```python
from build123d import *

# Parameters (mm, degrees)
SKETCH1_R           = 14.2875
BOSS_EXTRUDE1_DEPTH = 6.35
SKETCH2_R           = 3.3782
CUT_EXTRUDE1_DEPTH  = 7.35
CHAMFER1_SIZE       = 3.175


with BuildPart() as part:
    # Sketch1 → Boss-Extrude1 (new body)
    with BuildSketch(Plane(origin=(0, 0, 0), x_dir=(0, 0, -1), z_dir=(1, 0, 0))):
        with BuildLine():
            Line((0, 0), (0, 25.4))
            Line((0, 25.4), (28.110381264, 81.266707127))
            ThreePointArc((28.110381264, 81.266707127), (50.8, 95.25), (73.489618736, 81.266707127))
            Line((73.489618736, 81.266707127), (101.6, 25.4))
            Line((101.6, 25.4), (101.6, 0))
            Line((101.6, 0), (0, 0))
        make_face()
        with Locations((50.8, 69.85)):
            Circle(SKETCH1_R, mode=Mode.SUBTRACT)
    extrude(amount=BOSS_EXTRUDE1_DEPTH)

    # Sketch2 → Cut-Extrude1 (cut, through all)
    with BuildSketch(Plane(origin=(6.35, 0, 0), x_dir=(0, 0, -1), z_dir=(1, 0, 0))):
        with Locations((12.7, 12.7)):
            Circle(SKETCH2_R)
        with Locations((50.8, 12.7)):
            Circle(SKETCH2_R)
        with Locations((88.9, 12.7)):
            Circle(SKETCH2_R)
    extrude(amount=-CUT_EXTRUDE1_DEPTH, mode=Mode.SUBTRACT)

    # Chamfer1
    chamfer1_edges = [part.edges().sort_by_distance(p)[0] for p in [
        (3.175, 0, 0),
        (3.175, 0, -101.6),
    ]]
    chamfer(chamfer1_edges, length=CHAMFER1_SIZE)


solid = part.part
```
Input: part model. Units: mm. Frame: model coordinates. Round coordinates to 2 decimals unless told otherwise and drop trailing zeros. Loops run counter-clockwise (first coordinate to the right, second up) from the corner with the lowest first, then second, coordinate; pieces in that order, holes last. Notation, with made-up numbers: (-32.5, -34.75) - (-28.5, -34.75) arc R18 ccw to (-28.5, -0.75) - close; hole circle Ø10 at (16, -39). An arc over 180 degrees is marked (long way). One line per item, written item: value. Start each with the question number.
(1) Contact query for flat-ended pins moving along their axis: P1, Ø3, axis at x = 1, z = -57.5, coming from the +Y side; P2, Ø2, axis at x = 4.5, z = -35.5, coming from the +Y side. Output: stop coordinate, or through.
(2) Section C-C, the plane x = 5. Count the separate pieces of the cut face and the enclosed holes in it, plus the area to 3 significant figures.
(3) Ray query, line 1 (Y direction, x = 3.25, z = -50.8); line 2 (Y direction, x = 1.75, z = -88); line 3 (Y direction, x = 3, z = -53.5). Return the intervals inside material, ascending. Write a range as [from, to].
(4) Section A-A, the plane y = 12.7. Return loops of the section in (x, z), plus the area to 3 significant figures.
(5) Draft query along Y for faces 1 (the flat face through (3, 14, 0)), 2 (the cylindrical face through (3.131, 84.016, -48.94)), 3 (the flat face through (3.131, 1.565, -1.61)), 4 (the cylindrical face through (3.219, 10.644, -10.019)). Return one class per face: +Y half, -Y half, draft (parallel to the pull), parting line (faces both ways), or undercut.
(6) Section B-B, the plane z = -50.8. Return loops of the section in (x, y).
(7) Section D-D, the plane y = 69.85. Return loops of the section in (x, z), plus the area to 3 significant figures.
Results below:
1. P1: y = 94.71
1. P2: y = 90.84
2. separate pieces: 1
2. enclosed holes: 4
2. area: 6,380 mm^2
3. line 1: [0, 9.32], [16.08, 55.56], [84.14, 95.25]
3. line 2: [0, 9.44], [15.96, 52.43]
3. line 3: [0, 10.67], [14.73, 55.82], [83.88, 95.11]
4. outline: (0, -101.6) - (6.35, -101.6) - (6.35, -92.28) - (0, -92.28) - close; (0, -85.52) - (6.35, -85.52) - (6.35, -54.18) - (0, -54.18) - close; (0, -47.42) - (6.35, -47.42) - (6.35, -16.08) - (0, -16.08) - close; (0, -9.32) - (6.35, -9.32) - (6.35, 0) - (0, 0) - close
4. area: 516 mm^2
5. face 1: draft
5. face 2: undercut
5. face 3: -Y half
5. face 4: undercut
6. outline: (0, 0) - (6.35, 0) - (6.35, 9.32) - (0, 9.32) - close; (0, 16.08) - (6.35, 16.08) - (6.35, 55.56) - (0, 55.56) - close; (0, 84.14) - (6.35, 84.14) - (6.35, 95.25) - (0, 95.25) - close
7. outline: (0, -79.23) - (6.35, -79.23) - (6.35, -65.09) - (0, -65.09) - close; (0, -36.51) - (6.35, -36.51) - (6.35, -22.37) - (0, -22.37) - close
7. area: 180 mm^2
